```python
from build123d import *

# Parameters (mm, degrees)
SKETCH1_W           = 30
SKETCH1_H           = 34
BOSS_EXTRUDE1_DEPTH = 16.7
SKETCH2_W           = 10.7
SKETCH2_H           = 23
CUT_EXTRUDE1_DEPTH  = 49.94129136
HOLE1_D             = 4.4
HOLE2_D             = 4.4
HOLE3_D             = 4.4
HOLE4_D             = 4.4
HOLE5_D             = 4.4
HOLE6_D             = 4.4
HOLE7_D             = 8
HOLE7_DEPTH         = 34
RIB1_REACH          = 43.476
SKETCH17_WALL_W     = 108.907794566
SKETCH17_WALL_H     = 5


with BuildPart() as part:
    # Sketch1 → Boss-Extrude1 (new body)
    with BuildSketch(Plane.XY.offset(-8.3)):
        with Locations((-26.5, 12.5)):
            Rectangle(SKETCH1_W, SKETCH1_H)
    extrude(amount=-BOSS_EXTRUDE1_DEPTH)

    # Sketch2 → Cut-Extrude1 (cut, through all)
    with BuildSketch(Plane.ZY.offset(41.5)):
        with Locations((-19.65, 18)):
            Rectangle(SKETCH2_W, SKETCH2_H)
    extrude(amount=-CUT_EXTRUDE1_DEPTH, mode=Mode.SUBTRACT)

    # Hole1 (through all)
    with Locations(Plane(origin=(0, 0, -14.3), x_dir=(-1, 0, 0), z_dir=(0, 0, -1))):
        with Locations((16.5, 12.25)):
            Hole(HOLE1_D / 2)

    # Hole2 (through all)
    with Locations(Plane(origin=(0, 0, -14.3), x_dir=(-1, 0, 0), z_dir=(0, 0, -1))):
        with Locations((36.5, 12.25)):
            Hole(HOLE2_D / 2)

    # Hole3 (through all)
    with Locations(Plane(origin=(0, 0, -14.3), x_dir=(-1, 0, 0), z_dir=(0, 0, -1))):
        with Locations((36.5, 24.75)):
            Hole(HOLE3_D / 2)

    # Hole4 (through all)
    with Locations(Plane(origin=(0, 0, -14.3), x_dir=(-1, 0, 0), z_dir=(0, 0, -1))):
        with Locations((16.5, 24.75)):
            Hole(HOLE4_D / 2)

    # Hole5 (through all)
    with Locations(Plane(origin=(0, 0, -25), x_dir=(-1, 0, 0), z_dir=(0, 0, -1))):
        with Locations((36, 1)):
            Hole(HOLE5_D / 2)

    # Hole6 (through all)
    with Locations(Plane.XY.offset(-8.3)):
        with Locations((-17, 1)):
            Hole(HOLE6_D / 2)

    # Hole7
    with Locations(Plane.XZ.offset(4.5)):
        with Locations((-26.5, -25)):
            Hole(HOLE7_D / 2, depth=HOLE7_DEPTH)

    # Sketch17 wall → Rib1 (add, up to next)
    with BuildSketch(Plane(origin=(-26.5, 18, -17.65), x_dir=(0, -0.960093451224, -0.279679396661), z_dir=(0, -0.279679396661, 0.960093451224)), mode=Mode.PRIVATE) as rib1_sk1:
        Rectangle(SKETCH17_WALL_W, SKETCH17_WALL_H)
    rib1_tool1 = extrude(rib1_sk1.sketch, amount=RIB1_REACH, mode=Mode.PRIVATE) - part.part
    add(rib1_tool1.solids().sort_by_distance((-26.5, 18, -17.65))[0])


solid = part.part
```
CAD build for the part. Positions are in the model's coordinates, mm. A direction names the side the tool comes from. Coordinates: 2 decimals unless noted, no trailing zeros. Order: outer loops, then holes, each group sorted by start corner. A loop starts at its lowest first (then second) coordinate and runs counter-clockwise, first axis right, second up.
(1) Saw through at C-C, the plane x = -36.5. Write the cut outline in (y, z).
Solution:
outline: (-4.5, -25) - (-1.14, -25) - (-1.14, -8.3) - (-4.5, -8.3) - close; (3.14, -25) - (6.5, -25) - (6.5, -14.3) - (10.05, -14.3) - (10.05, -8.3) - (3.14, -8.3) - close; (14.45, -14.3) - (22.55, -14.3) - (22.55, -8.3) - (14.45, -8.3) - close; (26.95, -14.3) - (29.5, -14.3) - (29.5, -8.3) - (26.95, -8.3) - close
(2) Pin check, flat tips, straight feed: pin 1 Ø3.5 at (x, y) = (-16.5, 12.25) entering from +Z; pin 2 Ø7 at (x, y) = (-36.5, 24.75) entering from -Z; pin 3 Ø1 at (x, z) = (-38, -16) entering from +Y; pin 4 Ø2 at (x, y) = (-26.5, 14) entering from -Z. Stop position of each tip, or through.
Solution:
pin 1: passes through
pin 2: stops at z = -14.3
pin 3: stops at y = 6.5
pin 4: stops at z = -19.11
(3) Mould opens along Y. For faces 1 (the face through (-36, 6.5, -20)), 2 (the face through (-38.7, 12.3, -11.3)), 3 (the face through (-27, -4.5, -17)) say: released by +Y, released by -Y, zero draft, split by the parting line, or undercut.
Solution:
face 1: released by +Y
face 2: undercut
face 3: released by -Y
(4) Drill centre lines: L1, parallel to Y at x = -36.5, z = -10.8; L2, parallel to Y at x = -36, z = -16; L3, parallel to X at y = -1, z = -15.75. Where is each one in solid material? Low to high.
Solution:
L1: y = -4.5 to -1.14, 3.14 to 10.05, 14.45 to 22.55, 26.95 to 29.5
L2: y = -4.5 to -1.2, 3.2 to 6.5
L3: x = -41.5 to -36.92, -35.08 to -17.92, -16.08 to -11.5
(5) Saw through at D-D, the plane z = -19. Write the cut outline in (x, y), and give its area (3 significant figures).
Solution:
outline: (-41.5, -4.5) - (-11.5, -4.5) - (-11.5, 6.5) - (-24, 6.5) - (-24, 13.37) - (-29, 13.37) - (-29, 6.5) - (-41.5, 6.5) - close; hole circle Ø4.4 at (-36, 1); hole circle Ø4.4 at (-17, 1)
area: 334 mm2
(6) Saw through at A-A, the plane y = 1. Write the cut outline in (x, z), and give its area (3 significant figures).
Solution:
outline: (-41.5, -25) - (-38.2, -25) - (-38.2, -8.3) - (-41.5, -8.3) - close; (-33.8, -25) - (-30.5, -25) arc R4 cw to (-22.5, -25) - (-19.2, -25) - (-19.2, -8.3) - (-33.8, -8.3) - close; (-14.8, -25) - (-11.5, -25) - (-11.5, -8.3) - (-14.8, -8.3) - close
area: 329 mm2
(7) Saw through at B-B, the plane z = -12. Write the cut outline in (x, y).
Solution:
outline: (-41.5, -4.5) - (-11.5, -4.5) - (-11.5, 29.5) - (-41.5, 29.5) - close; hole circle Ø4.4 at (-36.5, 12.25); hole circle Ø4.4 at (-36.5, 24.75); hole circle Ø4.4 at (-36, 1); hole circle Ø4.4 at (-17, 1); hole circle Ø4.4 at (-16.5, 12.25); hole circle Ø4.4 at (-16.5, 24.75)
(8) Which spindle directions (+Z, -Z, +X, -X, +Y, -Y) get a long thin tool onto all of the face, cutting with end or side? Do faces 4 (the face through (-15.48, 22.8, -11.26)), 5 (the face through (-35, 18, -14.3)), 6 (the face through (-18, 18, -14.3)). Say none if no direction does.
Solution:
face 4: +Z, -Z
face 5: -Z, -X, +Y
face 6: -Z, +X, +Y
